from build123d import *

# Parameters (mm, degrees)
SKETCH1_R               = 9.525
BOSS_EXTRUDE1_DEPTH     = 12.5
CUT_EXTRUDE1_REACH      = 14.5
SKETCH2_R               = 3
SKETCH3_R               = 9.525
BOSS_EXTRUDE2_DEPTH     = 13.3375
SKETCH4_W               = 12.7
SKETCH4_H               = 12.3375
CUT_EXTRUDE2_DEPTH      = 13.3375
CUT_EXTRUDE2_DEPTH_BACK = 13.3375
SKETCH5_R               = 2.413
CUT_EXTRUDE4_DEPTH      = 13.3375


with BuildPart() as part:
    # Sketch1 → Boss-Extrude1 (new body)
    with BuildSketch(Plane(origin=(0, 0, 0), x_dir=(1, 0, 0), z_dir=(0, 1, 0))):
        Circle(SKETCH1_R)
    extrude(amount=BOSS_EXTRUDE1_DEPTH)

    # Sketch2 → Cut-Extrude1 (cut, up to next)
    with BuildSketch(Plane(origin=(0, 12.5, 0), x_dir=(1, 0, 0), z_dir=(0, 1, 0)), mode=Mode.PRIVATE) as cut_extrude1_sk1:
        Circle(SKETCH2_R)
    cut_extrude1_tool1 = extrude(cut_extrude1_sk1.sketch, amount=-CUT_EXTRUDE1_REACH, mode=Mode.PRIVATE) & part.part
    add(cut_extrude1_tool1.solids().sort_by_distance((0, 12.5, 0))[0], mode=Mode.SUBTRACT)

    # Sketch3 → Boss-Extrude2 (add)
    with BuildSketch(Plane(origin=(0, 12.5, 0), x_dir=(1, 0, 0), z_dir=(0, 1, 0))):
        Circle(SKETCH3_R)
    extrude(amount=BOSS_EXTRUDE2_DEPTH)

    # Sketch4 → Cut-Extrude2 (cut, two sides)
    with BuildSketch(Plane.XY) as cut_extrude2_sk:
        with Locations((0, 19.66875)):
            Rectangle(SKETCH4_W, SKETCH4_H)
    extrude(amount=CUT_EXTRUDE2_DEPTH, mode=Mode.SUBTRACT)
    extrude(cut_extrude2_sk.sketch, amount=-CUT_EXTRUDE2_DEPTH_BACK, mode=Mode.SUBTRACT)

    # Sketch5 → Cut-Extrude4 (cut)
    with BuildSketch(Plane.XY):
        with Locations((0, 9.944)):
            Circle(SKETCH5_R)
    extrude(amount=-CUT_EXTRUDE4_DEPTH, mode=Mode.SUBTRACT)


solid = part.part
Design review of the part built by this model. Coordinates are the model's own, in mm. A direction names the side the tool comes from. Round coordinates to 2 decimals unless told otherwise and drop trailing zeros. Write each loop counter-clockwise with the first axis right and the second up, starting at its lowest first coordinate (ties: lowest second). Pieces come first, ordered by that corner, then holes. Notation, with made-up numbers: (-34.75, 3.5) - (5.25, 3.5) arc R31 ccw to (5.25, 35.5) - close; hole circle Ø3 at (-8, 15.25). An arc over 180 degrees is marked (long way). Return JSON: item names as keys, results as strings. Group by question number.
Item 1: For probe 1 along X at (y, z) = (8.75, 0) (3 decimals); probe 2 along Y at (x, z) = (0, -7), list the stretches that pass through material, from the lowest coordinate up. Write a range as [from, to].
Item 2: We need section A-A on x = 0. Write out the cut boundary in (y, z) (3 decimals), and give its area (3 significant figures).
Item 3: We need section C-C on y = 15.25. Write out the cut boundary in (x, z) (3 decimals).
Item 4: The part is to be moulded in two halves that separate along Z. For faces 5 (the face through (0, 12.5, 0)), 6 (the face through (-7.559, 9.867, 5.796)), 7 (the face through (-2.3, 0, -2.3)), say which applies: pulls with the +Z half, pulls with the -Z half, needs draft (parallel to the pull), parting line crosses it, or undercut.
Item 5: We need section D-D on z = -6.5. Write out the cut boundary in (x, y), and give its area (3 significant figures).
Item 6: Machinability: for faces 1 (the face through (-8, 25.838, 0)), 2 (the face through (-0.65, 6.34, 2.93)), 3 (the face through (2.3, 10.67, -5.6)), 4 (the face through (6.35, 20, 0)), which of the approach directions +Z, -Z, +X, -X, +Y, -Y give a long, thin tool a straight path to every point of the face, cutting with its end or side? Answer none if there is none.
Item 7: Insertion check: P1, Ø8, axis at y = 18, z = -4.5, coming from the -X side; P2, Ø4, axis at x = -5.5, y = 23, coming from the +Z side; P3, Ø1.5, axis at y = 22.5, z = 6.5, coming from the -X side. Each pin has a flat end and moves straight along its axis. Give the tip position at first contact, or say it passes through.
Model answer:
{
 "1": {"probe 1": "x = [-9.525, -3], [3, 9.525]", "probe 2": "y = [0, 7.53], [12.36, 13.5]"},
 "2": {"outline": "(0, -9.525) - (7.531, -9.525) - (7.531, -3) - (0, -3) - close; (0, 3) - (12.5, 3) - (12.5, -3) - (12.357, -3) - (12.357, -9.525) - (13.5, -9.525) - (13.5, 9.525) - (0, 9.525) - close", "area": "151 mm²"},
 "3": {"outline": "(-6.35, -7.1) - (-6.35, 7.1) arc R9.525 ccw to start; (6.35, -7.1) arc R9.525 ccw to (6.35, 7.1) - close"},
 "4": {"face 5": "undercut", "face 6": "parting line crosses it", "face 7": "needs draft"},
 "5": {"outline": "(-6.96, 0) - (6.96, 0) - (6.96, 25.84) - (6.35, 25.84) - (6.35, 13.5) - (-6.35, 13.5) - (-6.35, 25.84) - (-6.96, 25.84) - close; hole circle Ø4.83 at (0, 9.94)", "area": "185 mm²"},
 "6": {"face 1": "+Z, -Z, +X, -X, +Y", "face 2": "-Y", "face 3": "-Z", "face 4": "+Z, -Z, +Y"},
 "7": {"P1": "stops at x = -9.51", "P2": "stops at z = 7.1", "P3": "stops at x = -7.59"}
}
